Source: CAD feature listing. Evaluate the final solid. Frame: model axes, mm. A direction names the side the tool comes from. Give positions to 0.01 mm unless a question says otherwise; leave off trailing zeros. Loops run counter-clockwise (first coordinate to the right, second up) from the corner with the lowest first, then second, coordinate; pieces in that order, holes last. Notation, with made-up numbers: (4.5, 35) -> (26.5, 35) arc R21 ccw to (26.5, 60) -> close; hole circle Ø11 at (86.5, -14.75). An arc over 180 degrees is marked (long way). Put each result on its own line as item: value.
Autodesk Inventor part; units mm, degrees
ref_plane "YZ Plane" through (0, 0, 0) normal (1, 0, 0) x (0, 1, 0)
ref_plane "XZ Plane" through (0, 0, 0) normal (0, 1, 0) x (-1, 0, 0)
ref_plane "XY Plane" through (0, 0, 0) normal (0, 0, 1) x (1, 0, 0)
sketch "Sketch1" plane through (0, 0, 0) normal (0, 1, 0) x (-1, 0, 0)
  line L0 (0, 0) -> (80, 0)
  line L1 (80, 0) -> (80, -5)
  line L2 (80, -5) -> (0, -5)
  line L3 (0, -5) -> (0, 0)
  dimension "d0" = 5
  dimension "d1" = 80
extrude "Extrusion1" add sketch "Sketch1" along normal blind 3
sketch "Sketch2" plane through (0, 3, 0) normal (0, 1, 0) x (1, 0, 0)
  line L0 (0, 3.825) -> (-80, 3.825)
  line L1 (-80, 3.825) -> (-80, 1.175)
  line L2 (-80, 1.175) -> (0, 1.175)
  line L3 (0, 1.175) -> (0, 3.825)
  line L4 (0, 3.825) -> (-80, 1.175) construction
  line L5 (-80, 3.825) -> (0, 1.175) construction
  line L6 (0, 0) -> (0, 5)
  line L7 (-80, 5) -> (-80, 0)
  point P0 (-40, 2.5)
  point P1 (0, 2.5)
  point P2 (0, 2.5)
  dimension "d4" = 2.65
extrude "Extrusion2" add sketch "Sketch2" along normal blind 4.826
sketch "Sketch3" plane through (0, 0, 0) normal (1, 0, 0) x (0, 0, -1)
  line L0 (5, 7.826) -> (0, 7.826)
  line L1 (0, 7.826) -> (0, 15.326)
  line L2 (0, 15.326) -> (5, 15.326)
  line L3 (5, 15.326) -> (5, 7.826)
  line L4 (1.175, 7.826) -> (3.825, 7.826)
  line L5 (5, 0) -> (5, 3)
  line L6 (0, 0) -> (0, 3)
  line L7 (0, 15.326) -> (-5, 15.326)
  line L8 (-5, 15.326) -> (-5, 12.326)
  line L9 (-5, 12.326) -> (0, 12.326)
  line L10 (0, 12.326) -> (0, 15.326)
  dimension "d7" = 7.5
  dimension "d8" = 3
  dimension "d9" = 5
extrude "Extrusion3" add sketch "Sketch3" against normal up to surface (80 mm away)
fillet "Fillet1" radius 1.5 3 edges at (-40, 15.326, -5) (-40, 15.326, 5) (-40, 12.326, 5)
fillet "Fillet2" radius 1.5 2 edges at (-40, 0, 0) (-40, 0, -5)
properties part number "Rails"
(1) Line query: probe 1 along Y at (x, z) = (-4, 3); probe 2 along Y at (x, z) = (-50.5, -0.25); probe 3 along Z at (x, y) = (-43.5, 4.25) (3 decimals). Output: solid intervals per line, ascending. Write a range as from..to.
Calculated:
probe 1: y = 12.33..15.33
probe 2: y = 0.67..3, 7.83..15.33
probe 3: z = -3.825..-1.175
(2) Section B-B on y = 11.5. Return loops of the section in (x, z), then the cut area to 3 significant figures.
Calculated:
outline: (-80, -5) -> (0, -5) -> (0, 0) -> (-80, 0) -> close
area: 400 mm²
(3) Draft query along Y for faces 1 (the cylindrical face through (-40.56, 14.9, -4.55)), 2 (the flat face through (-39, 11, -5)), 3 (the flat face through (-39, 12.326, 2)), 4 (the flat face through (-39, 5, -3.825)). Return one class per face: released by +Y, released by -Y, zero draft, split by the parting line, or undercut.
Calculated:
face 1: released by +Y
face 2: zero draft
face 3: released by -Y
face 4: undercut
(4) Section C-C on z = 1.25. Return loops of the section in (x, y).
Calculated:
outline: (-80, 12.33) -> (0, 12.33) -> (0, 15.33) -> (-80, 15.33) -> close
(5) First-contact query: P1, Ø5, axis at x = -54, y = 11, coming from the +Z side; P2, Ø1.1, axis at x = -54, z = 1.5, coming from the -Y side; P3, Ø1.5, axis at x = -56.5, y = 2, coming from the +Z side. Flat tips, straight axial feed; report the tip coordinate or a pass-through.
Calculated:
P1: stops at z = 4.96
P2: stops at y = 12.33
P3: stops at z = 0
(6) Reachability of faces 5 (the flat face through (-39, 2, 0)), 6 (the flat face through (-41, 5, -1.175)), 7 (the flat face through (0, 9, -1)) from +Z, -Z, +X, -X, +Y, -Y: full face, straight path, thin tool, end or side. Return the list, or none.
Calculated:
face 5: +Z, +X, -X, -Y
face 6: +Z, +X, -X
face 7: +Z, -Z, +X, +Y, -Y
